Build history of the part. All positions in model axes, mm. A direction names the side the tool comes from. Give positions to 0.01 mm unless a question says otherwise; leave off trailing zeros. Order: outer loops, then holes, each group sorted by start corner. A loop starts at its lowest first (then second) coordinate and runs counter-clockwise, first axis right, second up. Notation, with made-up numbers: (8, 42.5) - (38, 42.5) arc R24 ccw to (38, 78.5) - close; hole circle Ø9 at (-35.5, 18). An arc over 180 degrees is marked (long way). Use a Markdown table: item, result. Add a question column.
(1) Slice it at C-C (y = 9.5). Write the cut outline in (x, z), then the cut area to 3 significant figures.
(2) Slice it at A-A (y = 15). Write the cut outline in (x, z), then the cut area to 3 significant figures.
(3) Flat gauge pins, fed straight in: pin 1 (1.5 mm diameter, centred on y = 24.5, z = 14.5, fed in from +X); pin 2 (4 mm diameter, centred on y = 5, z = 6, fed in from +X); pin 3 (5 mm diameter, centred on x = 16.5, y = 9, fed in from +Z). Where does each tip first touch, or does it go through?
(4) Slice it at B-B (z = 5.5). Write the cut outline in (x, y).
(5) Wall check: line 1 (Z direction, x = 23.75, y = 12.5); line 2 (Z direction, x = 23.25, y = 15); line 3 (Y direction, x = 11.75, z = 8). Give the ranges that are in metal, low to high.
(6) Slice it at D-D (z = 16.5). Write the cut outline in (x, y).
(7) Mould opens along X. For faces 4 (the face through (25.5, 14.9, 4.5)), 5 (the face through (2.31, 4.2, 4.11)), 6 (the face through (18.958, 19.97, 18.842)) say: +X half, -X half, draft (parallel to the pull), parting line (faces both ways), or undercut.
(8) Which spindle directions (+Z, -Z, +X, -X, +Y, -Y) get a long thin tool onto all of the face, cutting with end or side? Do faces 1 (the face through (13, 15, 7)), 2 (the face through (0, 18, 11)), 3 (the face through (25, 21, 11)). Say none if no direction does.
from build123d import *

# Parameters (mm, degrees)
CYLINDER016027_R            = 3
CYLINDER016027_DEPTH        = 3
CYLINDER016026_R            = 1.65
CYLINDER016026_DEPTH        = 15
CYLINDER016025_R            = 2
CYLINDER016025_DEPTH        = 15
BOX031_W                    = 10
BOX031_H                    = 10
BOX031_DEPTH                = 42
BOX032_W                    = 10
BOX032_H                    = 10
BOX032_DEPTH                = 42
BOX029_W                    = 17
BOX029_H                    = 20
BOX029_DEPTH                = 32
FILLET007_R                 = 3
FILLET008_R                 = 1
BOX025_W                    = 25
BOX025_H                    = 26
BOX025_DEPTH                = 15
FILLET008003_R              = 7
CHAMFER016016008004014_SIZE = 0.4
BOX026_W                    = 2
BOX026_H                    = 7.8
BOX026_DEPTH                = 15
CHAMFER016016008004011_SIZE = 1
CHAMFER016016008004015_SIZE = 0.4


with BuildPart() as cylinder041:
    # Cylinder016027 → Cylinder016027 (new body)
    with BuildSketch(Plane(origin=(21, 15, 11.5), x_dir=(0, 0, -1), z_dir=(1, 0, 0))):
        Circle(CYLINDER016027_R)
    extrude(amount=CYLINDER016027_DEPTH)


with BuildPart() as cylinder040:
    # Cylinder016026 → Cylinder016026 (new body)
    with BuildSketch(Plane(origin=(20.5, 15, 11.5), x_dir=(0, 0, -1), z_dir=(1, 0, 0))):
        Circle(CYLINDER016026_R)
    extrude(amount=CYLINDER016026_DEPTH)


with BuildPart() as cylinder039:
    # Cylinder016025 → Cylinder016025 (new body)
    with BuildSketch(Plane(origin=(-2, 15, 11.5), x_dir=(0, 0, -1), z_dir=(1, 0, 0))):
        Circle(CYLINDER016025_R)
    extrude(amount=CYLINDER016025_DEPTH)


with BuildPart() as cube031:
    # Box031 → Box031 (new body)
    with BuildSketch(Plane(origin=(21.5, 22.5, 0), x_dir=(1, 0, 0), z_dir=(0, 0, 1))):
        with Locations((5, 5)):
            Rectangle(BOX031_W, BOX031_H)
    extrude(amount=BOX031_DEPTH)


with BuildPart() as cube032:
    # Box032 → Box032 (new body)
    with BuildSketch(Plane(origin=(18.5, 19.5, 0), x_dir=(1, 0, 0), z_dir=(0, 0, 1))):
        with Locations((5, 5)):
            Rectangle(BOX032_W, BOX032_H)
    extrude(amount=BOX032_DEPTH)


with BuildPart() as inner_cut:
    # Box029 → Box029 (new body)
    with BuildSketch(Plane(origin=(5, 5, 4), x_dir=(1, 0, 0), z_dir=(0, 0, 1))):
        with Locations((8.5, 10)):
            Rectangle(BOX029_W, BOX029_H)
    extrude(amount=BOX029_DEPTH)

    # Cut010011008009003005: cut Cube032
    add(cube032.part, mode=Mode.SUBTRACT)

    # Fillet007
    fillet007_edges = [inner_cut.edges().sort_by_distance(p)[0] for p in [
        (5, 5, 20),
        (5, 25, 20),
        (22, 5, 20),
        (18.5, 25, 20),
    ]]
    fillet(fillet007_edges, radius=FILLET007_R)

    # Fillet008
    fillet008_edges = [inner_cut.edges().sort_by_distance(p)[0] for p in [
        (18.5, 19.5, 20),
        (22, 19.5, 20),
    ]]
    fillet(fillet008_edges, radius=FILLET008_R)


with BuildPart() as inner_cut_1:
    # Fillet008 placement: moved
    add(inner_cut.part.moved(Location((0, 0, 3))))


with BuildPart() as chamfer016016008004014:
    # Box025 → Box025 (new body)
    with BuildSketch(Plane(origin=(0, 2, 4), x_dir=(1, 0, 0), z_dir=(0, 0, 1))):
        with Locations((12.5, 13)):
            Rectangle(BOX025_W, BOX025_H)
    extrude(amount=BOX025_DEPTH)

    # Cut010011008009003009: cut inner-cut
    add(inner_cut_1.part, mode=Mode.SUBTRACT)

    # Fillet008003
    fillet008003_edges = [chamfer016016008004014.edges().sort_by_distance(p)[0] for p in [
        (0, 2, 11.5),
        (0, 28, 11.5),
    ]]
    fillet(fillet008003_edges, radius=FILLET008003_R)

    # Cut010011008009003010: cut Cube031
    add(cube031.part, mode=Mode.SUBTRACT)

    # Chamfer016016008004014
    chamfer016016008004014_edges = [chamfer016016008004014.edges().sort_by_distance(p)[0] for p in [
        (0, 15, 19),
        (0, 15, 4),
        (2.050253, 25.949747, 19),
        (14.25, 28, 19),
        (21.5, 25.25, 19),
        (23.25, 22.5, 19),
        (25, 12.25, 19),
        (16, 2, 19),
        (2.050253, 4.050253, 19),
        (18.5, 21.25, 19),
        (18.792893, 19.792893, 19),
        (17.62132, 24.12132, 19),
        (20.25, 19.5, 19),
        (11.75, 25, 19),
        (21.707107, 19.207107, 19),
        (5.87868, 24.12132, 19),
        (22, 13.25, 19),
        (5, 15, 19),
        (21.12132, 5.87868, 19),
        (5.87868, 5.87868, 19),
        (13.5, 5, 19),
        (2.050253, 4.050253, 4),
        (2.050253, 25.949747, 4),
        (14.25, 28, 4),
        (21.5, 25.25, 4),
        (23.25, 22.5, 4),
        (25, 12.25, 4),
        (16, 2, 4),
        (21.5, 28, 11.5),
    ]]
    chamfer(chamfer016016008004014_edges, length=CHAMFER016016008004014_SIZE)


with BuildPart() as obj1:
    # Box026 → Box026 (new body)
    with BuildSketch(Plane(origin=(24, 11.1, 4), x_dir=(1, 0, 0), z_dir=(0, 0, 1))):
        with Locations((1, 3.9)):
            Rectangle(BOX026_W, BOX026_H)
    extrude(amount=BOX026_DEPTH)

    # Chamfer016016008004011
    chamfer016016008004011_edges = [obj1.edges().sort_by_distance(p)[0] for p in [
        (26, 15, 19),
        (26, 15, 4),
    ]]
    chamfer(chamfer016016008004011_edges, length=CHAMFER016016008004011_SIZE)

    # Fusion018007003006: union Chamfer016016008004014
    add(chamfer016016008004014.part)

    # Cut010011008009003011: cut Cylinder039
    add(cylinder039.part, mode=Mode.SUBTRACT)

    # Chamfer016016008004015
    chamfer016016008004015_edges = [obj1.edges().sort_by_distance(p)[0] for p in [
        (0, 15, 13.5),
    ]]
    chamfer(chamfer016016008004015_edges, length=CHAMFER016016008004015_SIZE)

    # Cut010011008009003012: cut Cylinder040
    add(cylinder040.part, mode=Mode.SUBTRACT)

    # Cut010011008009003013: cut Cylinder041
    add(cylinder041.part, mode=Mode.SUBTRACT)


solid = obj1.part
Solution:
| question | item | result |
|---|---|---|
| 1 | outline | (0, 4.4) - (0.4, 4) - (24.6, 4) - (25, 4.4) - (25, 18.6) - (24.6, 19) - (22.4, 19) - (22, 18.6) - (22, 7) - (5, 7) - (5, 18.6) - (4.6, 19) - (0.4, 19) - (0, 18.6) - close |
| 1 | area | 171 mm2 |
| 2 | outline | (0, 4.4) - (0.4, 4) - (25, 4) - (26, 5) - (26, 9.85) - (24, 9.85) - (24, 8.5) - (22, 8.5) - (22, 7) - (5, 7) - (5, 9.5) - (0.4, 9.5) - (0, 9.1) - close; (0, 13.9) - (0.4, 13.5) - (5, 13.5) - (5, 18.6) - (4.6, 19) - (0.4, 19) - (0, 18.6) - close; (22, 14.5) - (24, 14.5) - (24, 13.15) - (26, 13.15) - (26, 18) - (25, 19) - (22.4, 19) - (22, 18.6) - close |
| 2 | area | 146 mm2 |
| 3 | pin 1 | x = 21.5 |
| 3 | pin 2 | x = 25 |
| 3 | pin 3 | z = 7 |
| 4 | outline | (0, 9) arc R7 ccw to (7, 2) - (25, 2) - (25, 11.1) - (26, 11.1) - (26, 18.9) - (25, 18.9) - (25, 22.5) - (21.5, 22.5) - (21.5, 27.6) - (21.1, 28) - (7, 28) arc R7 ccw to (0, 21) - close |
| 5 | line 1 | 4 to 9.84, 13.16 to 19 |
| 5 | line 2 | 4 to 8.5, 14.5 to 19 |
| 5 | line 3 | 2 to 5, 25 to 28 |
| 6 | outline | (0, 9) arc R7 ccw to (7, 2) - (25, 2) - (25, 11.1) - (26, 11.1) - (26, 18.9) - (25, 18.9) - (25, 22.5) - (21.5, 22.5) - (21.5, 27.6) - (21.1, 28) - (7, 28) arc R7 ccw to (0, 21) - close; hole (5, 8) arc R3 ccw to (8, 5) - (19, 5) arc R3 ccw to (22, 8) - (22, 18.5) arc R1 ccw to (21, 19.5) - (19.5, 19.5) arc R1 cw to (18.5, 20.5) - (18.5, 22) arc R3 ccw to (15.5, 25) - (8, 25) arc R3 ccw to (5, 22) - close |
| 7 | face 4 | +X half |
| 7 | face 5 | -X half |
| 7 | face 6 | undercut |
| 8 | face 1 | +Z |
| 8 | face 2 | +Z, -Z, -X, +Y, -Y |
| 8 | face 3 | +Z, -Z, +X, +Y |
